from build123d import *

# Parameters (mm, degrees)
SKETCH1_R          = 16.75
EXTRUDE1_DEPTH     = 1
SKETCH3_W          = 3
SKETCH3_H          = 19.5
EXTRUDE4_DEPTH     = 4
SKETCH4_W          = 2
SKETCH4_H          = 19.5
EXTRUDE5_DEPTH     = 2
SKETCH5_R          = 1.5
CUT_EXTRUDE1_DEPTH = 2


with BuildPart() as part:
    # Sketch1 → Extrude1 (new body)
    with BuildSketch(Plane.XY):
        Circle(SKETCH1_R)
    extrude(amount=EXTRUDE1_DEPTH)

    # Sketch3 → Extrude4 (add)
    with BuildSketch(Plane.XY.offset(1)):
        with Locations((6.5, 0)):
            Rectangle(SKETCH3_W, SKETCH3_H)
        Rectangle(SKETCH3_W, SKETCH3_H)
        with Locations((-6.5, 0)):
            Rectangle(SKETCH3_W, SKETCH3_H)
    extrude(amount=EXTRUDE4_DEPTH)

    # Sketch4 → Extrude5 (add)
    with BuildSketch(Plane.XY):
        with Locations((6.5, 0)):
            Rectangle(SKETCH4_W, SKETCH4_H)
        with Locations((-6.5, 0)):
            Rectangle(SKETCH4_W, SKETCH4_H)
        Rectangle(SKETCH4_W, SKETCH4_H)
    extrude(amount=-EXTRUDE5_DEPTH)

    # Sketch5 → Cut-Extrude1 (cut)
    with BuildSketch(Plane.XY):
        with Locations((-3.25, 6.25)):
            Circle(SKETCH5_R)
        with Locations((3.25, -6.262393856)):
            Circle(SKETCH5_R)
    extrude(amount=CUT_EXTRUDE1_DEPTH, mode=Mode.SUBTRACT)


solid = part.part
The model under review builds one solid part; all positions refer to its coordinate system, in mm. A direction names the side the tool comes from. Round coordinates to 2 decimals unless told otherwise and drop trailing zeros. Order: outer loops, then holes, each group sorted by start corner. A loop starts at its lowest first (then second) coordinate and runs counter-clockwise, first axis right, second up. Notation, with made-up numbers: (-13.5, 69) -> (23.5, 69) arc R26 cw to (23.5, 93) -> close; hole circle Ø2 at (70, -1). An arc over 180 degrees is marked (long way). Use CSV: the item, a comma, the result in double quotes. Start each with the question number.
(1) Consider section C-C on x = -3.25. Write out the cut boundary in (y, z), and give its area (3 significant figures).
(2) Consider section A-A on z = -1.25. Write out the cut boundary in (x, y), and give its area (3 significant figures).
(3) Tool access review of faces 1 (the face through (5, 0, 3)), 2 (the face through (-7, 9.75, 3)), 3 (the face through (0, -9.75, 3)): name each direction out of +Z, -Z, +X, -X, +Y, -Y from which nothing blocks a thin tool from reaching the whole face with its end or side.
(4) Wall thickness on probe 1 along X at (y, z) = (-9, 2); probe 2 along X at (y, z) = (9, -1); probe 3 along Z at (x, y) = (4, -1.5): over which ranges is each line inside the solid? List them lowest first. Write a range as from..to.
(5) Consider section B-B on y = 0. Write out the cut boundary in (x, z), and give its area (3 significant figures).
(6) Mouldability with a two-part tool opening along X and no side actions: class faces 4 (the face through (7.5, 0, -1)), 5 (the face through (0, 9.75, -1)), 6 (the face through (-1.5, 0, 3)) as pulls with the +X half, pulls with the -X half, needs draft (parallel to the pull), parting line crosses it, or undercut.
(7) Insertion check: pin 1 (1.2 mm diameter, centred on y = 4, z = 3.5, fed in from +X); pin 2 (1 mm diameter, centred on x = 3, y = -11.5, fed in from -Z); pin 3 (0.6 mm diameter, centred on y = -2.5, z = -0.5, fed in from +X); pin 4 (1 mm diameter, centred on x = -3.5, z = 4, fed in from -Y). Each pin has a flat end and moves straight along its axis. Give the tip position at first contact, or say it passes through.
Responses:
1,outline,"(-16.43, 0) -> (4.75, 0) -> (4.75, 1) -> (-16.43, 1) -> close; (7.75, 0) -> (16.43, 0) -> (16.43, 1) -> (7.75, 1) -> close"
1,area,"29.9 mm²"
2,outline,"(-7.5, -9.75) -> (-5.5, -9.75) -> (-5.5, 9.75) -> (-7.5, 9.75) -> close; (-1, -9.75) -> (1, -9.75) -> (1, 9.75) -> (-1, 9.75) -> close; (5.5, -9.75) -> (7.5, -9.75) -> (7.5, 9.75) -> (5.5, 9.75) -> close"
2,area,"117 mm²"
3,face 1,"+Z, +Y, -Y"
3,face 2,"+Z, +X, -X, +Y"
3,face 3,"+Z, +X, -X, -Y"
4,probe 1,"-8..-5, -1.5..1.5, 5..8"
4,probe 2,"-7.5..-5.5, -1..1, 5.5..7.5"
4,probe 3,"0..1"
5,outline,"(-16.75, 0) -> (-7.5, 0) -> (-7.5, -2) -> (-5.5, -2) -> (-5.5, 0) -> (-1, 0) -> (-1, -2) -> (1, -2) -> (1, 0) -> (5.5, 0) -> (5.5, -2) -> (7.5, -2) -> (7.5, 0) -> (16.75, 0) -> (16.75, 1) -> (8, 1) -> (8, 5) -> (5, 5) -> (5, 1) -> (1.5, 1) -> (1.5, 5) -> (-1.5, 5) -> (-1.5, 1) -> (-5, 1) -> (-5, 5) -> (-8, 5) -> (-8, 1) -> (-16.75, 1) -> close"
5,area,"81.5 mm²"
6,face 4,"pulls with the +X half"
6,face 5,"needs draft"
6,face 6,"undercut"
7,pin 1,"x = 8"
7,pin 2,"z = 0"
7,pin 3,"x = 7.5"
7,pin 4,"through"
